Input: part model. Units: mm. Frame: model coordinates. Face numbers are marked on the shaded views. Coordinates: 2 decimals unless noted, no trailing zeros. Order: outer loops, then holes, each group sorted by start corner. A loop starts at its lowest first (then second) coordinate and runs counter-clockwise, first axis right, second up. Notation, with made-up numbers: (61.25, 68) - (76.25, 68) arc R11 cw to (76.25, 85) - close; hole circle Ø2 at (-9.75, 48.25). An arc over 180 degrees is marked (long way). One line per question, with ' | ' between items.
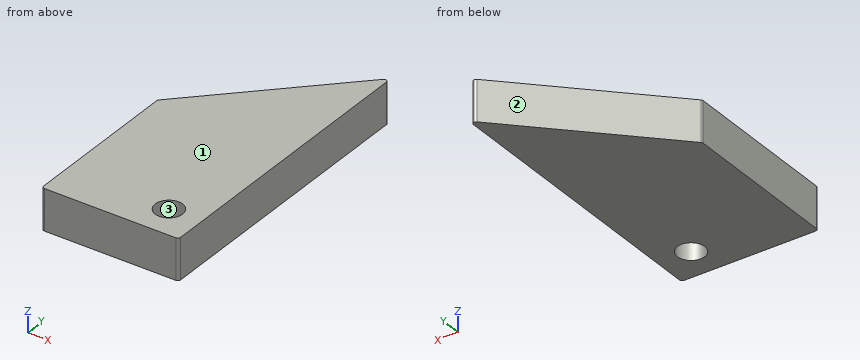
from build123d import *

# Parameters (mm, degrees)
SCHIZZO1_R                   = 5
ESTRUSIONE_ESTRUSIONE1_DEPTH = 15
RACCORDO1_R                  = 1


with BuildPart() as part:
    # Schizzo1 → Estrusione-Estrusione1 (new body)
    with BuildSketch(Plane.XY):
        Polygon((0, 0), (0, 110), (-50, 60), (-50, 0), align=None)
        with Locations((-12, 12)):
            Circle(SCHIZZO1_R, mode=Mode.SUBTRACT)
    extrude(amount=ESTRUSIONE_ESTRUSIONE1_DEPTH)

    # Raccordo1
    raccordo1_edges = [part.edges().sort_by_distance(p)[0] for p in [
        (-50, 0, 7.5),
        (-50, 60, 7.5),
        (0, 110, 7.5),
        (0, 0, 7.5),
    ]]
    fillet(raccordo1_edges, radius=RACCORDO1_R)


solid = part.part
Item 1: Section A-A on y = 12. Return the cut outline in (x, z), and give its area (3 significant figures).
Data:
outline: (-50, 0) - (-17, 0) - (-17, 15) - (-50, 15) - close; (-7, 0) - (0, 0) - (0, 15) - (-7, 15) - close | area: 600 mm^2
Item 2: Section C-C on x = -12. Return the cut outline in (y, z), and give its area (3 significant figures).
Data:
outline: (0, 0) - (7, 0) - (7, 15) - (0, 15) - close; (17, 0) - (98, 0) - (98, 15) - (17, 15) - close | area: 1,320 mm^2
Item 3: Section B-B on z = 13.75. Return the cut outline in (x, y), and give its area (3 significant figures).
Data:
outline: (-50, 1) arc R1 ccw to (-49, 0) - (-1, 0) arc R1 ccw to (0, 1) - (0, 107.59) arc R1 ccw to (-1.71, 108.29) - (-49.71, 60.29) arc R1 ccw to (-50, 59.59) - close; hole circle Ø10 at (-12, 12) | area: 4,170 mm^2
Item 4: Contact query for flat-ended pins moving along their axis: P1, Ø4, axis at x = -30, z = 8, coming from the +Y side; P2, Ø4, axis at x = -41, z = 8, coming from the +Y side; P3, Ø9, axis at x = -12, y = 12, coming from the -Z side; P4, Ø4, axis at x = -11, z = 1.5, coming from the +Y side. Output: stop coordinate, or through.
Data:
P1: y = 82 | P2: y = 71 | P3: through | P4: y = 101
Item 5: Draft query along X for the marked faces 1, 2 and 3. Return one class per face: released by +X, released by -X, zero draft, split by the parting line, or undercut.
Data:
face 1: zero draft | face 2: released by -X | face 3: undercut
Item 6: Ray query, line 1 (Y direction, x = -12, z = 8); line 2 (X direction, y = 13.5, z = 8.25); line 3 (Y direction, x = -5, z = 1). Return the intervals inside material, ascending.
Data:
line 1: 0 to 7, 17 to 98 | line 2: -50 to -16.77, -7.23 to 0 | line 3: 0 to 105
Item 7: Section D-D on x = -29. Return the cut outline in (y, z), and give its area (4 significant figures).
Data:
outline: (0, 0) - (81, 0) - (81, 15) - (0, 15) - close | area: 1,215 mm^2
